Check sheet for the modelled part. Datum: model origin and axes. Units: mm. Round coordinates to 2 decimals unless told otherwise and drop trailing zeros. Write each loop counter-clockwise with the first axis right and the second up, starting at its lowest first coordinate (ties: lowest second). Pieces come first, ordered by that corner, then holes. Notation, with made-up numbers: (19, -28) -> (60, -28) arc R13 ccw to (60, -19) -> close; hole circle Ø5 at (-21.75, 87.5). An arc over 180 degrees is marked (long way). Put each result on its own line as item: value. Start each with the question number.
from build123d import *

# Parameters (mm, degrees)
ESQUISSE4_R                  = 1.5
ESQUISSE5_R                  = 3
BOSS_EXTRU_1_DEPTH           = 10
ENL_V_MAT_EXTRU_1_DEPTH      = 1009.974851124
ENL_V_MAT_EXTRU_1_DEPTH_BACK = 1009.974851124
ESQUISSE6_R                  = 2


with BuildPart() as part:
    # Balayage1: sweep along a path in Esquisse3
    with BuildLine(Plane.XY) as balayage1_path:
        Line((-993, -170), (-993, 0))
        Line((-993, 0), (0, 0))
        Line((0, 0), (0, 86))
        Line((0, 86), (72, 86))
    # Esquisse4 → Balayage1 (sweep)
    with BuildSketch(Plane(origin=(-993, -170, 0), x_dir=(1, 0, 0), z_dir=(0, 1, 0))):
        Circle(ESQUISSE4_R)
    sweep(path=balayage1_path.line, transition=Transition.RIGHT)

    # Esquisse5 → Boss.-Extru.1 (add, symmetric)
    with BuildSketch(Plane.XY):
        Circle(ESQUISSE5_R)
        with Locations((72, 86)):
            Circle(ESQUISSE5_R)
    extrude(amount=BOSS_EXTRU_1_DEPTH, both=True)

    # Esquisse6 → Enlèv. mat.-Extru.1 (cut, two sides: drawn at the far end of the back side and taken through both)
    with BuildSketch(Plane.XY.offset(-ENL_V_MAT_EXTRU_1_DEPTH_BACK)):
        with Locations((72, 86)):
            Circle(ESQUISSE6_R)
        Circle(ESQUISSE6_R)
    extrude(amount=ENL_V_MAT_EXTRU_1_DEPTH + ENL_V_MAT_EXTRU_1_DEPTH_BACK, mode=Mode.SUBTRACT)

    # Esquisse7 → Révolution1 (revolve)
    with BuildSketch(Plane.XY):
        with BuildLine():
            Line((-996, -170), (-990, -170))
            ThreePointArc((-990, -170), (-993, -173), (-996, -170))
        make_face()
    revolve(axis=Axis((-996, -170, 0), (1, 0, 0)))


solid = part.part
1. Section check B-B, the plane y = -105.5. Enter the section's corners in (x, z), then the cut area to 3 significant figures.
2. Section check C-C, the plane x = -96.5. Enter the section's corners in (y, z), then the cut area to 3 significant figures.
3. Material ranges on L1, parallel to Y at x = 72, z = 4; L2, parallel to X at y = 86, z = -3.25; L3, parallel to X at y = 0, z = -3.75, recorded low to high. Write a range as [from, to].
4. Section check A-A, the plane z = 6.25. Enter the section's corners in (x, y), then the cut area to 3 significant figures.
5. Gauge pin test, flat ends, axial feed: P1, Ø2, axis at y = -8.5, z = 1, coming from the -X side; P2, Ø6, axis at y = -122.5, z = 2.5, coming from the +X side; P3, Ø6, axis at y = 26.5, z = -1, coming from the -X side. Record the tip position at first contact, or that the pin passes through.
Reply:
1. outline: circle Ø3 at (-993, 0)
1. area: 7.07 mm2
2. outline: circle Ø3 at (0, 0)
2. area: 7.07 mm2
3. L1: y = [83, 84], [88, 89]
3. L2: x = [69, 70], [74, 75]
3. L3: x = [-3, -2], [2, 3]
4. outline: circle Ø6 at (0, 0); circle Ø6 at (72, 86); hole circle Ø4 at (0, 0); hole circle Ø4 at (72, 86)
4. area: 31.4 mm2
5. P1: stops at x = -994.5
5. P2: stops at x = -991.5
5. P3: stops at x = -1.5
